Can you work these out from the model? Positions are in its coordinate system, mm. A direction names the side the tool comes from. Give positions to 0.01 mm unless a question says otherwise; leave off trailing zeros. Loops run counter-clockwise (first coordinate to the right, second up) from the corner with the lowest first, then second, coordinate; pieces in that order, holes last.
from build123d import *

# Parameters (mm, degrees)
F0_R      = 7
F0_R_2    = 4.5
F0_W      = 25
F0_H      = 20
F1_DEPTH  = 10
F2_W      = 25
F2_H      = 15
F2_W_2    = 12
F2_R      = 7
F2_R_2    = 4.5
F3_DEPTH  = 3
F4_W      = 30
F4_H      = 25
F5_DEPTH  = 5
F6_W      = 25
F6_H      = 20
F7_DEPTH  = 5
F8_R      = 1.75
F8_R_2    = 2.1
F9_DEPTH  = 25
F10_R     = 2.1
F11_DEPTH = 6
F12_W     = 20
F12_H     = 100
F12_H_2   = 104.976
F13_DEPTH = 25
F14_R     = 10.6
F14_R_2   = 2.1
F14_R_3   = 10.5
F15_DEPTH = 25
F16_W     = 45
F16_H     = 8
F17_DEPTH = 10
F18_R     = 2.1
F19_DEPTH = 6.85


with BuildPart() as f1:
    # F0 (on Top) → F1 (new body)
    with BuildSketch(Plane.XY):
        Polygon((-52.5, -98.8), (-40, -123.8), (-15, -123.8), (15, -123.8), (40, -123.8), (52.5, -98.8), (65, -98.8), (65, -73.8), (115, 26.2), (115, 46.2), (40, 46.2), (40, 36.2), (-40, 36.2), (-40, 46.2), (-115, 46.2), (-115, 26.2), (-65, -73.8), (-65, -98.8), align=None)
        Polygon((20, -98.8), (-20, -98.8), (0, -30), align=None, mode=Mode.SUBTRACT)
        Polygon((-80, 6.2), (-40, 6.2), (-40, -73.8), align=None, mode=Mode.SUBTRACT)
        with Locations((-75, 31.2)):
            Circle(F0_R, mode=Mode.SUBTRACT)
        Polygon((40, -73.8), (40, 6.2), (80, 6.2), align=None, mode=Mode.SUBTRACT)
        Circle(F0_R_2, mode=Mode.SUBTRACT)
        with Locations((75, 31.2)):
            Circle(F0_R, mode=Mode.SUBTRACT)
        with Locations((-27.5, -133.8)):
            Rectangle(F0_W, F0_H)
        with Locations((27.5, -133.8)):
            Rectangle(F0_W, F0_H)
    extrude(amount=F1_DEPTH)

    # F2 (on face) → F3 (join)
    with BuildSketch(Plane.XY.offset(10)):
        with Locations((-20.5, -7.5)):
            Rectangle(F2_W, F2_H)
        with Locations((20.5, -7.5)):
            Rectangle(F2_W, F2_H)
        with Locations((82.5, -7.5)):
            Rectangle(F2_W_2, F2_H)
        with Locations((-82.5, -7.5)):
            Rectangle(F2_W_2, F2_H)
        Circle(F2_R)
        Circle(F2_R_2, mode=Mode.SUBTRACT)
    extrude(amount=F3_DEPTH)

    # F4 (on face) → F5 (cut)
    with BuildSketch(Plane(origin=(0, 0, 0), x_dir=(1, 0, 0), z_dir=(0, 0, -1))):
        with Locations((0, 111.3)):
            Rectangle(F4_W, F4_H)
    extrude(amount=-F5_DEPTH, mode=Mode.SUBTRACT)

    # F6 (on face) → F7 (cut)
    with BuildSketch(Plane.XY.offset(10)):
        with Locations((-27.5, -133.8)):
            Rectangle(F6_W, F6_H)
        with Locations((27.5, -133.8)):
            Rectangle(F6_W, F6_H)
    extrude(amount=-F7_DEPTH, mode=Mode.SUBTRACT)

    # F8 (on face) → F9 (cut)
    with BuildSketch(Plane.XY.offset(10)):
        with Locations((-32, -137.8)):
            Circle(F8_R)
        with Locations((-23, -129.8)):
            Circle(F8_R)
        with Locations((23, -137.8)):
            Circle(F8_R)
        with Locations((32, -129.8)):
            Circle(F8_R)
        with Locations((-8, -116.8)):
            Circle(F8_R_2)
        with Locations((8, -116.8)):
            Circle(F8_R_2)
        with Locations((0, -105.8)):
            Circle(F8_R_2)
    extrude(amount=-F9_DEPTH, mode=Mode.SUBTRACT)

    # F10 (on face) → F11 (cut)
    with BuildSketch(Plane.XY.offset(13)):
        with Locations((-82.5, -7.5)):
            Circle(F10_R)
        with Locations((-27, -7.5)):
            Circle(F10_R)
        with Locations((27, -7.5)):
            Circle(F10_R)
        with Locations((82.5, -7.5)):
            Circle(F10_R)
        with Locations((-14, -7.5)):
            Circle(F10_R)
        with Locations((14, -7.5)):
            Circle(F10_R)
    extrude(amount=-F11_DEPTH, mode=Mode.SUBTRACT)

    # F12 (on face) → F13 (cut)
    with BuildSketch(Plane.XY.offset(10)):
        with Locations((-105, -3.8)):
            Rectangle(F12_W, F12_H)
        with Locations((105, -6.288)):
            Rectangle(F12_W, F12_H_2)
    extrude(amount=-F13_DEPTH, mode=Mode.SUBTRACT)

    # F14 (on face) → F15 (cut)
    with BuildSketch(Plane.XY.offset(10)):
        with Locations((-75, 31.2)):
            Circle(F14_R)
        with Locations((-63.686292, 42.513708)):
            Circle(F14_R_2)
        with Locations((-86.313708, 42.513708)):
            Circle(F14_R_2)
        with Locations((-86.313708, 19.886292)):
            Circle(F14_R_2)
        with Locations((-63.686292, 19.886292)):
            Circle(F14_R_2)
        with Locations((63.686292, 42.513708)):
            Circle(F14_R_2)
        with Locations((63.686292, 19.886292)):
            Circle(F14_R_2)
        with Locations((86.313708, 42.513708)):
            Circle(F14_R_2)
        with Locations((86.313708, 19.886292)):
            Circle(F14_R_2)
        with Locations((75, 31.2)):
            Circle(F14_R_3)
    extrude(amount=-F15_DEPTH, mode=Mode.SUBTRACT)

    # F16 (on face) → F17 (join)
    with BuildSketch(Plane.XY.offset(10)):
        with Locations((-72.5, 50.2)):
            Rectangle(F16_W, F16_H)
        with Locations((72.5, 50.2)):
            Rectangle(F16_W, F16_H)
    extrude(amount=-F17_DEPTH)

    # F18 (on face) → F19 (cut)
    with BuildSketch(Plane(origin=(0, 0, 0), x_dir=(1, 0, 0), z_dir=(0, 0, -1))):
        Polygon((4.116549, 6.5), (-4.116549, 6.5), (-7.19, 0), (-4.116549, -6.5), (4.116549, -6.5), (7.19, 0), align=None)
        with Locations((-20, 0)):
            Circle(F18_R)
        with Locations((20, 0)):
            Circle(F18_R)
    extrude(amount=-F19_DEPTH, mode=Mode.SUBTRACT)


solid = f1.part
(1) Please list where these lines run through material, in increasing order: probe 1 along X at (y, z) = (-12, 10.75); probe 2 along X at (y, z) = (31.5, 4); probe 3 along Y at (x, z) = (-86.5, 9).
Returned:
probe 1: x = -88.5 to -76.5, -33 to -8, 8 to 33, 76.5 to 88.5
probe 2: x = -95 to -85.6, -64.4 to 64.5, 85.5 to 95
probe 3: y = -30.8 to 17.79, 21.98 to 40.42, 44.61 to 54.2
(2) Thinking about a two-plate mould opening in Y: for faces 5 (the flat face through (15, -122, 2)), 6 (the flat face through (45, 46.2, 5)), 7 (the flat face through (-5.675, 3.205, 3.377)), which applies, pulls with the +Y half, pulls with the -Y half, needs draft (parallel to the pull), parting line crosses it, or undercut?
Returned:
face 5: needs draft
face 6: pulls with the +Y half
face 7: undercut
(3) Which directions (+Z, -Z, +X, -X, +Y, -Y) give clear straight access to the entire face, cutting with the end or side of a thin tool? Please do faces 1 (the cylindrical face through (26.727, -5.418, 10.042)), 2 (the flat face through (-40, -33, 5)), 3 (the flat face through (1.5, -4.42, 6.85)), 4 (the flat face through (-28, -134, 5)).
Returned:
face 1: +Z
face 2: +Z, -Z
face 3: -Z
face 4: +Z, +X, -X, -Y
(4) Will these pins go through, and if not, where does the flat tip stop? P1, Ø4, axis at x = -86.31, y = 19.89, coming from the +Z side; P2, Ø2.5, axis at x = -21, z = 12, coming from the +Y side; P3, Ø6, axis at x = -37.5, z = 8.5, coming from the -Y side; P4, Ø3, axis at y = -28, z = 5.5, coming from the -X side.
Returned:
P1: passes through
P2: stops at y = 0
P3: stops at y = -123.8
P4: stops at x = -88.65
(5) Suppose I cut it at B-B on y = -101. List the corners of the cut face in (x, z) for me.
Returned:
outline: (-51.4, 0) - (-15, 0) - (-15, 5) - (15, 5) - (15, 0) - (51.4, 0) - (51.4, 10) - (-51.4, 10) - close
(6) Suppose I cut it at A-A on x = 57.5. List the corners of the cut face in (y, z) for me, plus the area to 3 significant figures.
Returned:
outline: (-98.8, 0) - (-38.8, 0) - (-38.8, 10) - (-98.8, 10) - close; (6.2, 0) - (54.2, 0) - (54.2, 10) - (6.2, 10) - close
area: 1,080 mm2
(7) Suppose I cut it at C-C on x = -57. List the corners of the cut face in (y, z) for me, plus the area to 3 significant figures.
Returned:
outline: (-98.8, 0) - (-39.8, 0) - (-39.8, 10) - (-98.8, 10) - close; (6.2, 0) - (54.2, 0) - (54.2, 10) - (6.2, 10) - close
area: 1,070 mm2
